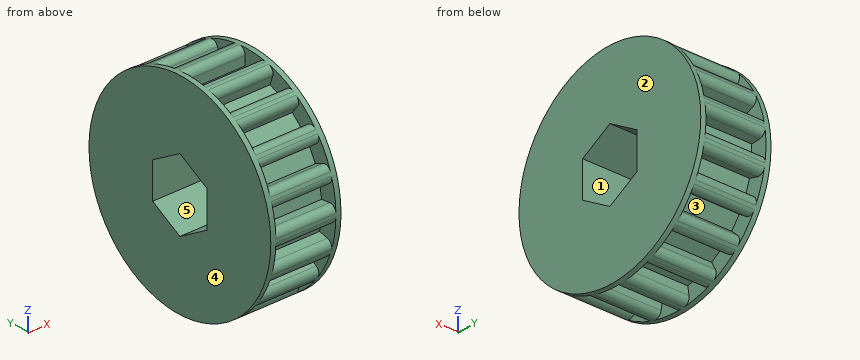
from build123d import *

# Parameters (mm, degrees)
REVOLVE1_START           = -5.5
REVOLVE1_OUTLINE_R       = 15.875
REVOLVE1_OUTLINE_R_2     = 3.175
REVOLVE1_DEPTH           = 11
CUT_EXTRUDE1_START       = -0.79375
CUT_EXTRUDE1_DEPTH       = 9.4125
FILLET1_R                = 1
CIRPATTERN1_COUNT        = 19
FILLET1_OF_CIRPATTERN1_R = 1
CUT_EXTRUDE2_DEPTH       = 26.000624992


# Read off the part's stored shape, not the designer's step: Revolve1
with BuildPart() as part:
    # Revolve1 outline → Revolve1 (new body)
    with BuildSketch(Plane.YZ.offset(REVOLVE1_START)):
        Circle(REVOLVE1_OUTLINE_R)
        Circle(REVOLVE1_OUTLINE_R_2, mode=Mode.SUBTRACT)
    extrude(amount=REVOLVE1_DEPTH)

    # Sketch2 → Cut-Extrude1 (cut)
    with BuildSketch(Plane(origin=(5.5, 0, 0), x_dir=(0, 0, -1), z_dir=(1, 0, 0)).offset(CUT_EXTRUDE1_START)):
        Polygon((-1.091836735, 13.375), (1.091836735, 13.375), (1.5, 18.375), (-1.5, 18.375), align=None)
    cut_extrude1 = extrude(amount=-CUT_EXTRUDE1_DEPTH, mode=Mode.SUBTRACT)

    # Fillet1
    fillet1_edges = [part.edges().sort_by_distance(p)[0] for p in [
        (0, 15.822368276, -1.2916219),
        (0, 15.822368276, 1.2916219),
    ]]
    fillet(fillet1_edges, radius=FILLET1_R)

    # CirPattern1: Cut-Extrude1 ×19 about axis
    cirpattern1_axis = Axis((0, 0, 0), (1, 0, 0))
    for i in range(1, CIRPATTERN1_COUNT):
        add(cut_extrude1.rotate(cirpattern1_axis, i * 360 / CIRPATTERN1_COUNT), mode=Mode.SUBTRACT)

    # Fillet1 of CirPattern1
    fillet1_of_cirpattern1_edges = [part.edges().sort_by_distance(p)[0] for p in [
        (0, 15.384457666, 3.915876318),
        (0, 14.545679775, 6.359152844),
        (0, 13.279402352, 8.699028576),
        (0, 11.69274117, 10.737570904),
        (0, 9.735317743, 12.539506108),
        (0, 7.572712628, 13.952406547),
        (0, 5.136260397, 15.021133583),
        (0, 2.632063171, 15.655282446),
        (0, -0.01939046, 15.874988158),
        (0, -2.593811173, 15.661665576),
        (0, -5.172940059, 15.008541439),
        (0, -7.538605828, 13.970864224),
        (0, -9.765921337, 12.515686375),
        (0, -11.666475568, 10.766102954),
        (0, -13.300613505, 8.66656249),
        (0, -14.530101657, 6.394667375),
        (0, -15.393977818, 3.878282085),
        (0, -15.819165773, 1.330270363),
        (0, -15.819165773, -1.330270363),
        (0, -15.393977818, -3.878282085),
        (0, -14.530101657, -6.394667375),
        (0, -13.300613505, -8.66656249),
        (0, -11.666475568, -10.766102954),
        (0, -9.765921337, -12.515686375),
        (0, -7.538605828, -13.970864224),
        (0, -5.172940059, -15.008541439),
        (0, -2.593811173, -15.661665576),
        (0, -0.01939046, -15.874988158),
        (0, 2.632063171, -15.655282446),
        (0, 5.136260397, -15.021133583),
        (0, 7.572712628, -13.952406547),
        (0, 9.735317743, -12.539506108),
        (0, 11.69274117, -10.737570904),
        (0, 13.279402352, -8.699028576),
        (0, 14.545679775, -6.359152844),
        (0, 15.384457666, -3.915876318),
    ]]
    fillet(fillet1_of_cirpattern1_edges, radius=FILLET1_OF_CIRPATTERN1_R)

    # Sketch3 → Cut-Extrude2 (cut, through all)
    with BuildSketch(Plane(origin=(5.5, 0, 0), x_dir=(0, 0, -1), z_dir=(1, 0, 0))):
        Polygon((5.499261314, 0), (2.749630657, 4.7625), (-2.749630657, 4.7625), (-5.499261314, 0), (-2.749630657, -4.7625), (2.749630657, -4.7625), align=None)
    extrude(amount=-CUT_EXTRUDE2_DEPTH, mode=Mode.SUBTRACT)


solid = part.part
Design review of the part built by this model. Coordinates are the model's own, in mm. Face numbers are marked on the shaded views. A direction names the side the tool comes from. Round coordinates to 2 decimals unless told otherwise and drop trailing zeros. Write each loop counter-clockwise with the first axis right and the second up, starting at its lowest first coordinate (ties: lowest second). Pieces come first, ordered by that corner, then holes. Notation, with made-up numbers: M 88.5,68 L 129.5,68 A29 ccw 129.5,94 Z; hole C 17.25,-24 d11. An arc over 180 degrees is marked long. One line per item, written item: value. Start each with the question number.
1. Draft analysis for pull direction Y (two halves, no side actions). For the marked faces 4 and 5, state which applies: pulls with the +Y half, pulls with the -Y half, needs draft (parallel to the pull), parting line crosses it, or undercut.
2. Take a section at A-A on z = 4.5. State the section outline as (x, y) points, then the cut area to 3 significant figures.
3. Clearance check with flat-ended pins moving along their axes: P1, Ø6, axis at x = -2.5, z = -8, coming from the -Y side; P2, Ø3, axis at x = -0.5, z = 9, coming from the -Y side; P3, Ø1.5, axis at x = 3.5, z = -5, coming from the +Y side. State where each tip first meets the part, or that it passes through.
4. To check wall thickness, follow probe 1 along X at (y, z) = (7, 11.5); probe 2 along Z at (x, y) = (3.75, -9); probe 3 along Z at (x, y) = (2.5, -4). State the ranges of each line that lie inside material, in increasing order. Write a range as from..to.
5. For the marked faces 1, 2 and 3, list the 3-axis set-ups (+Z, -Z, +X, -X, +Y, -Y) from which the entire face can be reached by the end or side of a thin tool; tool diameter is ignored.
Computed:
1. face 4: needs draft
1. face 5: undercut
2. outline: M -5.5,-15.22 L -4.71,-15.22 L -4.71,-15.14 L 4.71,-15.14 L 4.71,-15.22 L 5.5,-15.22 L 5.5,-1.73 L -5.5,-1.73 Z; M -5.5,1.73 L 5.5,1.73 L 5.5,15.22 L 4.71,15.22 L 4.71,12.6 L -4.71,12.6 L -4.71,15.22 L -5.5,15.22 Z
2. area: 271 mm²
3. P1: stops at y = -15.07
3. P2: stops at y = -12.89
3. P3: stops at y = 13.15
4. probe 1: x = -5.5..-4.71, 4.71..5.5
4. probe 2: z = -13.07..-11.53, -9.89..9.89, 11.53..13.07
4. probe 3: z = -15.36..-3.19, 3.19..15.36
5. face 1: +X, -X
5. face 2: +Z, -Z, +X, +Y, -Y
5. face 3: none
